Autodesk Inventor part; units mm, degrees
ref_plane "YZ Plane" through (0, 0, 0) normal (1, 0, 0) x (0, 1, 0)
ref_plane "XZ Plane" through (0, 0, 0) normal (0, 1, 0) x (-1, 0, 0)
ref_plane "XY Plane" through (0, 0, 0) normal (0, 0, 1) x (1, 0, 0)
sketch "Szkic1" plane through (0, 0, 0) normal (1, 0, 0) x (0, 1, 0)
  line L0 (0, 0) -> (0, 55)
  line L1 (0, 0) -> (-60, 0)
  line L2 (-60, 0) -> (0, 55)
  dimension "d0" = 55
  dimension "d1" = 60
extrude "Wyciągnięcie proste1" add sketch "Szkic1" along normal blind 150
sketch "Szkic2" plane through (0, -60, 0) normal (0, -0.6757246, 0.7371541) x (1, 0, 0)
  line L0 (0, 81.3941) -> (150, 81.3941)
  line L1 (55, 81.3941) -> (95, 81.3941)
  line L2 (95, 81.3941) -> (95, 65.3941)
  line L3 (95, 65.3941) -> (55, 65.3941)
  line L4 (55, 65.3941) -> (55, 81.3941)
  point P0 (0, 44.2292)
  dimension "d4" = 40
  dimension "d5" = 16
extrude "Wyciągnięcie proste2" cut sketch "Szkic2" against normal blind 15
sketch "Szkic3" plane through (0, -60, 0) normal (0, -0.6757246, 0.7371541) x (1, 0, 0)
  line L0 (55, 65.3941) -> (95, 65.3941)
  line L1 (95, 65.3941) -> (95, 59.3941)
  line L2 (95, 59.3941) -> (55, 59.3941)
  line L3 (55, 59.3941) -> (55, 65.3941)
  point P0 (0, 44.2292)
  dimension "d8" = 40
  dimension "d9" = 6
extrude "Wyciągnięcie proste3" cut sketch "Szkic3" against normal blind 15
sketch "Szkic4" plane through (0, -60, 0) normal (0, -0.6757246, 0.7371541) x (1, 0, 0)
  line L0 (55, 59.3941) -> (95, 59.3941)
  line L1 (95, 59.3941) -> (95, 53.3941)
  line L2 (95, 53.3941) -> (55, 53.3941)
  line L3 (55, 53.3941) -> (55, 59.3941)
  point P0 (0, 44.2292)
  dimension "d12" = 40
  dimension "d13" = 6
extrude "Wyciągnięcie proste4" cut sketch "Szkic4" against normal blind 15
properties part number "klin" material "Brąz, odlew"
For this review, take the finished solid that the model builds, in its own axes (mm). A direction names the side the tool comes from. Round coordinates to 2 decimals unless told otherwise and drop trailing zeros. Write each loop counter-clockwise with the first axis right and the second up, starting at its lowest first coordinate (ties: lowest second). Pieces come first, ordered by that corner, then holes. Notation, with made-up numbers: (48.25, 2.5) -> (73.25, 2.5) arc R12 cw to (73.25, 7.5) -> close; hole circle Ø3 at (33, 32). An arc over 180 degrees is marked (long way). One line per question, with ' | ' between items. Start each with the question number.
1) Machinability: for faces 1 (the flat face through (74.72, -5.18, 29.9)), 2 (the flat face through (74, 0, 27)), which of the approach directions +Z, -Z, +X, -X, +Y, -Y give a long, thin tool a straight path to every point of the face, cutting with its end or side? Answer none if there is none.
2) Add section B-B (x = 70). Write out the cut boundary in (y, z).
3) Wall thickness on line 1 along X through (y, z) = (-7.5, 30); line 2 along Y through (x, z) = (98.5, 37); line 3 along Y through (x, z) = (44.5, 51): over which ranges is each line inside the solid? List them lowest first.
4) For pin 1 Ø2 at (y, z) = (-35.5, 26.5) entering from -X; pin 2 Ø12 at (x, z) = (25, 18.5) entering from -Y, all flat-tipped, find the tip position at first contact; note any pin that passes through.
5) Add section D-D (y = -8). Write out the cut boundary in (x, z), and give its area (3 significant figures).
6) Add section C-C (z = 26.5). Write out the cut boundary in (x, y).
7) Add section A-A (z = 38.5). Write out the cut boundary in (x, y).
8) Mouldability with a two-part tool opening along X and no side actions: class faces 3 (the flat face through (150, -17, 16)), 4 (the flat face through (73.95, -30.42, 27.115)), 5 (the flat face through (0, -17, 16)), 6 (the flat face through (55, -8, 38)) as +X half, -X half, draft (parallel to the pull), parting line (faces both ways), or undercut.
Reported:
1) face 1: +Z | face 2: +Z, -Z, +X, -X, +Y
2) outline: (-60, 0) -> (0, 0) -> (0, 34.65) -> (-10.5, 25.02) -> (-20.64, 36.08) -> close
3) line 1: x = 0 to 55, 95 to 150 | line 2: y = -19.64 to 0 | line 3: y = -4.36 to 0
4) pin 1: passes through | pin 2: stops at y = -46.36
5) outline: (0, 0) -> (150, 0) -> (150, 47.67) -> (95, 47.67) -> (95, 27.32) -> (55, 27.32) -> (55, 47.67) -> (0, 47.67) -> close | area: 6,340 mm²
6) outline: (0, -31.09) -> (150, -31.09) -> (150, 0) -> (0, 0) -> close; hole (55, -11.86) -> (95, -11.86) -> (95, -8.89) -> (55, -8.89) -> close
7) outline: (0, -18) -> (55, -18) -> (55, 0) -> (0, 0) -> close; (95, -18) -> (150, -18) -> (150, 0) -> (95, 0) -> close
8) face 3: +X half | face 4: draft | face 5: -X half | face 6: undercut
